```python
from build123d import *

# Parameters (mm, degrees)
EXTRUDE1_DEPTH          = 4.5
CUT_EXTRUDE1_DEPTH      = 8
CUT_EXTRUDE1_DEPTH_BACK = 8
EXTRUDE2_DEPTH          = 6.00039994
CUT_EXTRUDE2_DEPTH      = 4
CUT_EXTRUDE2_DEPTH_BACK = 4
CUT_REVOLVE1_ANGLE      = 60
CUT_REVOLVE2_ANGLE      = 60
SKETCH9_R               = 2.48793
CUT_EXTRUDE3_DEPTH      = 7.00040004
FILLET4_R               = 0.25
SKETCH10_R              = 2.48793
EXTRUDE3_DEPTH          = 6.0004
SKETCH12_R              = 3.175
CUT_EXTRUDE4_DEPTH      = 7.00040004


with BuildPart() as part:
    # Sketch1 → Extrude1 (new body)
    with BuildSketch(Plane(origin=(0, 0, 0), x_dir=(1, 0, 0), z_dir=(0, 1, 0))):
        with BuildLine():
            Line((0, -8), (2.85, -8))
            ThreePointArc((2.85, -8), (3.557106781, -7.707106781), (3.85, -7))
            Line((3.85, -7), (3.85, 6.393551439))
            ThreePointArc((3.85, 6.393551439), (3.688791661, 6.938003962), (3.2571429, 7.306915911))
            ThreePointArc((3.2571429, 7.306915911), (1.66503344, 7.824810774), (0, 8))
            Line((0, 8), (-2.85, 8))
            ThreePointArc((-2.85, 8), (-3.557106781, 7.707106781), (-3.85, 7))
            Line((-3.85, 7), (-3.85, -6.393551439))
            ThreePointArc((-3.85, -6.393551439), (-3.688791661, -6.938003962), (-3.2571429, -7.306915911))
            ThreePointArc((-3.2571429, -7.306915911), (-1.66503344, -7.824810774), (0, -8))
        make_face()
    extrude(amount=EXTRUDE1_DEPTH)

    # Sketch2 → Cut-Extrude1 (cut, two sides)
    with BuildSketch(Plane.XY) as cut_extrude1_sk:
        Polygon((-4, 4.5), (-3.5, 4), (-3, 4.5), (-2.5, 4), (-2, 4.5), (-1.5, 4), (-1, 4.5), (-0.5, 4), (0, 4.5), (0.5, 4), (1, 4.5), (1.5, 4), (2, 4.5), (2.5, 4), (3, 4.5), (3.5, 4), (4, 4.5), (4, 5.5), (-4, 5.5), align=None)
    extrude(amount=CUT_EXTRUDE1_DEPTH, mode=Mode.SUBTRACT)
    extrude(cut_extrude1_sk.sketch, amount=-CUT_EXTRUDE1_DEPTH_BACK, mode=Mode.SUBTRACT)

    # Sketch3 → Extrude2 (add)
    with BuildSketch(Plane(origin=(0, 0, 0), x_dir=(1, 0, 0), z_dir=(0, 1, 0))):
        with BuildLine():
            Line((0.15, -3.85), (2.693303618, -3.85))
            ThreePointArc((2.693303618, -3.85), (3.511211473, -3.511211473), (3.85, -2.693303618))
            Line((3.85, -2.693303618), (3.85, -0.15))
            ThreePointArc((3.85, -0.15), (2.678427125, 2.678427125), (-0.15, 3.85))
            Line((-0.15, 3.85), (-2.85, 3.85))
            ThreePointArc((-2.85, 3.85), (-3.557106781, 3.557106781), (-3.85, 2.85))
            Line((-3.85, 2.85), (-3.85, 0.15))
            ThreePointArc((-3.85, 0.15), (-2.678427125, -2.678427125), (0.15, -3.85))
        make_face()
    extrude(amount=EXTRUDE2_DEPTH)

    # Sketch4 → Cut-Extrude2 (cut, two sides)
    with BuildSketch(Plane(origin=(0, 0, 0), x_dir=(0, 0, -1), z_dir=(1, 0, 0))) as cut_extrude2_sk:
        Polygon((-9, -1), (9, -1), (9, 4), (5, 0), (-5, 0), (-9, 4), align=None)
    extrude(amount=CUT_EXTRUDE2_DEPTH, mode=Mode.SUBTRACT)
    extrude(cut_extrude2_sk.sketch, amount=-CUT_EXTRUDE2_DEPTH_BACK, mode=Mode.SUBTRACT)

    # Sketch5 → Cut-Revolve1 (revolve, cut)
    with BuildSketch(Plane(origin=(0, 0, 0), x_dir=(0, 0, -1), z_dir=(1, 0, 0))):
        Polygon((0, -1), (-9, -1), (-9, 3), (-8, 3), (-5, 0), (0, 0), align=None)
    revolve(axis=Axis((0, 3, 0), (0, -1, 0)), revolution_arc=CUT_REVOLVE1_ANGLE, mode=Mode.SUBTRACT)

    # Sketch6 → Cut-Revolve2 (revolve, cut)
    with BuildSketch(Plane(origin=(0, 0, 0), x_dir=(0, 0, -1), z_dir=(1, 0, 0))):
        Polygon((0, 0), (5, 0), (8, 3), (9, 3), (9, -1), (0, -1), align=None)
    revolve(axis=Axis((0, -1, 0), (0, -1, 0)), revolution_arc=CUT_REVOLVE2_ANGLE, mode=Mode.SUBTRACT)

    # Sketch9 → Cut-Extrude3 (cut, through all)
    with BuildSketch(Plane(origin=(0, 6.00039994, 0), x_dir=(1, 0, 0), z_dir=(0, 1, 0))):
        Circle(SKETCH9_R)
    extrude(amount=-CUT_EXTRUDE3_DEPTH, mode=Mode.SUBTRACT)

    # Fillet4
    fillet4_edges = [part.edges().sort_by_distance(p)[0] for p in [
        (-2.678427125, 6.00039994, 2.678427125),
        (1.421651809, 6.00039994, 3.85),
        (3.511211473, 6.00039994, 3.511211473),
        (3.85, 6.00039994, 1.421651809),
        (2.678427125, 6.00039994, -2.678427125),
        (-1.5, 6.00039994, -3.85),
        (-3.557106781, 6.00039994, -3.557106781),
        (-3.85, 6.00039994, -1.5),
    ]]
    fillet(fillet4_edges, radius=FILLET4_R)

    # Sketch10 → Extrude3 (add)
    with BuildSketch(Plane(origin=(0, 6.00039994, 0), x_dir=(1, 0, 0), z_dir=(0, 1, 0))):
        Circle(SKETCH10_R)
    extrude(amount=-EXTRUDE3_DEPTH)

    # Sketch12 → Cut-Extrude4 (cut, through all)
    with BuildSketch(Plane(origin=(0, 6.00039994, 0), x_dir=(1, 0, 0), z_dir=(0, 1, 0))):
        Circle(SKETCH12_R)
    extrude(amount=-CUT_EXTRUDE4_DEPTH, mode=Mode.SUBTRACT)


solid = part.part
```
The model under review builds one solid part; all positions refer to its coordinate system, in mm. A direction names the side the tool comes from. Coordinates: 2 decimals unless noted, no trailing zeros. Write each loop counter-clockwise with the first axis right and the second up, starting at its lowest first coordinate (ties: lowest second). Pieces come first, ordered by that corner, then holes.
1) We need section A-A on y = 5. State the section outline as (x, z) points (3 decimals), then the cut area to 3 significant figures.
2) The part is to be moulded in two halves that separate along X. For faces 3 (the face through (3.663, 3.51, 7.583)), 4 (the face through (1, 5, 3.85)), 5 (the face through (-2, 2, -7)), 6 (the face through (-0.69, 3.04, 3.1)), say which applies: pulls with the +X half, pulls with the -X half, needs draft (parallel to the pull), parting line crosses it, or undercut.
3) Machinability: for faces 1 (the face through (1, 4, 8)), 2 (the face through (-2.709, 5.057, 2.647)), which of the approach directions +Z, -Z, +X, -X, +Y, -Y give a long, thin tool a straight path to every point of the face, cutting with its end or side? Answer none if there is none.
4) To check wall thickness, follow probe 1 along X at (y, z) = (3.25, 0) (3 decimals); probe 2 along Z at (x, y) = (0, 2) (3 decimals); probe 3 along X at (y, z) = (0.5, 1.5). State the ranges of each line that lie inside material, in increasing order.
5) Clearance check with flat-ended pins moving along their axes: pin 1 Ø1.9 at (x, y) = (1, 5.5) entering from +Z; pin 2 Ø1 at (x, y) = (2, 3) entering from -Z; pin 3 Ø1.5 at (x, z) = (-2.5, -6) entering from -Y. State where each tip first meets the part, or that it passes through.
6) We need section B-B on y = 1.25. State the section outline as (x, z) points (3 decimals), then the cut area to 3 significant figures.
Answer list:
1. outline: (-3.85, -2.85) arc R1 ccw to (-2.85, -3.85) - (-0.15, -3.85) arc R4 ccw to (3.85, 0.15) - (3.85, 2.693) arc R1.157 ccw to (2.693, 3.85) - (0.15, 3.85) arc R4 ccw to (-3.85, -0.15) - close; hole circle Ø6.35 at (0, 0)
1. area: 20.3 mm2
2. face 3: pulls with the +X half
2. face 4: undercut
2. face 5: needs draft
2. face 6: undercut
3. face 1: +Z, +X, -X, +Y, -Y
3. face 2: +Z, +Y
4. probe 1: x = -3.85 to -3.175, 3.175 to 3.85
4. probe 2: z = -7 to -3.175, 3.175 to 7
4. probe 3: x = -3.85 to -2.8, 2.8 to 3.85
5. pin 1: stops at z = 3.85
5. pin 2: stops at z = -7.86
5. pin 3: stops at y = 0.25
6. outline: (-3.85, -6.25) - (0, -6.25) arc R6.25 ccw to (3.85, -4.923) - (3.85, 6.25) - (0, 6.25) arc R6.25 ccw to (-3.85, 4.923) - close; hole circle Ø6.35 at (0, 0)
6. area: 61.3 mm2
